CAD build for the part. Positions are in the model's coordinates, mm. A direction names the side the tool comes from. Coordinates: 2 decimals unless noted, no trailing zeros. Write each loop counter-clockwise with the first axis right and the second up, starting at its lowest first coordinate (ties: lowest second). Pieces come first, ordered by that corner, then holes. Notation, with made-up numbers: M -13,47 L 30,47 A16 cw 30,55 Z; hole C 27,57.25 d5. An arc over 180 degrees is marked long. Put each result on its own line as item: value. Start each with the question number.
Autodesk Inventor part; units mm, degrees
ref_plane "YZ Plane" through (0, 0, 0) normal (1, 0, 0) x (0, 1, 0)
ref_plane "XZ Plane" through (0, 0, 0) normal (0, 1, 0) x (-1, 0, 0)
ref_plane "XY Plane" through (0, 0, 0) normal (0, 0, 1) x (1, 0, 0)
sketch "Boceto1" plane through (0, 0, 0) normal (0, 1, 0) x (-1, 0, 0)
  circle A0 centre (0, 0) radius 37
  dimension "d0" = 74
extrude "Extrusión1" add sketch "Boceto1" along normal blind 11
sketch "Boceto3" plane through (0, 0, 0) normal (0, -1, 0) x (1, 0, 0)
  circle A0 centre (0, 0) radius 8.25
  circle A1 centre (0, 8.25) radius 1.7
  circle A2 centre (8.25, 0) radius 1.7
  circle A3 centre (-8.25, 0) radius 1.7
  circle A4 centre (0, -8.25) radius 1.7
  dimension "d7" = 3.4
  dimension "d8" = 16.5
extrude "Extrusión3" cut sketch "Boceto3" against normal through all contours A0 A2 | A0 A2 | A1 A0 | A0 A1 | A4 A0 | A0 A4 | A3 A0 | A0 A3
sketch "Boceto5" plane through (0, 0, 0) normal (0, -1, 0) x (1, 0, 0)
  circle A0 centre (0, 0) radius 4.05
  dimension "d13" = 8.1
extrude "Extrusión5" cut sketch "Boceto5" against normal through all
sketch "Boceto8" plane through (0, 11, 0) normal (0, 1, 0) x (1, 0, 0)
  circle A0 centre (0, 0) radius 24.5
  circle A1 centre (0, 0) radius 37
  dimension "d25" = 49
  dimension "d26" = 74
extrude "Extrusión8" cut sketch "Boceto8" against normal blind 4
sketch "Boceto14" plane through (0, 7, 0) normal (0, 1, 0) x (1, 0, 0)
  circle A0 centre (0, 0) radius 28
  circle A1 centre (0, 28) radius 1.7
  circle A2 centre (-24.2487, 14) radius 1.7
  circle A3 centre (-24.2487, -14) radius 1.7
  circle A4 centre (0, -28) radius 1.7
  circle A5 centre (24.2487, -14) radius 1.7
  circle A6 centre (24.2487, 14) radius 1.7
  point P0 (-1.6992, -27.9484)
  point P1 (1.6992, -27.9484)
  dimension "d50" = 56
  dimension "d51" = 3.4
  dimension "d54" = 360
extrude "Extrusión12" cut sketch "Boceto14" against normal through all contours A6 A0 | A0 A6 | A5 A0 | A0 A5 | A1 A0 | A0 A1 | A4 A0 | A0 A4 | A2 A0 | A0 A2 | A3 A0 | A0 A3
sketch "Boceto15" plane through (0, 7, 0) normal (0, 1, 0) x (1, 0, 0)
  circle A0 centre (24.2487, 14) radius 1.7
  circle A1 centre (24.2487, 14) radius 3
  circle A2 centre (0, 28) radius 3
  circle A3 centre (-24.2487, 14) radius 3
  circle A4 centre (-24.2487, -14) radius 3
  circle A5 centre (0, -28) radius 3
  circle A6 centre (24.2487, -14) radius 3
  circle A7 centre (0, 0) radius 4.05
  circle A8 centre (0, 0) radius 32.5
  circle A9 centre (0, 0) radius 24.5
  dimension "d58" = 6
  dimension "d61" = 360
  dimension "d63" = 65
extrude "Extrusión13" cut sketch "Boceto15" against normal blind 3 contours A0 | A1 | A2 | A3 | A4 | A5 | A6 | A8
sketch "Boceto16" plane through (0, 11, 0) normal (0, 1, 0) x (1, 0, 0)
  circle A0 centre (0, 0) radius 4.05
  circle A1 centre (0, 0) radius 14.5
  circle A2 centre (0, 0) radius 37
  dimension "d66" = 29
extrude "Extrusión14" cut sketch "Boceto16" against normal blind 4 contours A2
equation "\"d1\" = Altura"
equation "\"Altura\" = 11"
properties part number "Joint - Primer segmento" material "Plastico PETG"
(1) Slice it at C-C, the plane z = 28. Write the cut outline in (x, y).
(2) Slice it at A-A, the plane z = 0. Write the cut outline in (x, y), then the cut area to 3 significant figures.
(3) Slice it at D-D, the plane x = -8.25. Write the cut outline in (y, z).
(4) Drill centre lines: line 1 (Z direction, x = 0, y = 3.05); line 2 (X direction, y = 6.75, z = -7.5); line 3 (Z direction, x = 0, y = 6). Where is each one in solid material? Low to high. Write a range as [from, to].
(5) Two-plate mould, pull along Z, no slides. Class faces 3 (the face through (-3, 11, -3)), 4 (the face through (6.691, 9.028, 12.864)), 5 (the face through (-0.37, 5.42, -9.91)): +Z half, -Z half, draft (parallel to the pull), parting line (faces both ways), or undercut.
(6) Drop flat-ended pins along their axis: pin 1 (3 mm diameter, centred on x = 8, z = 24, fed in from +Y); pin 2 (6 mm diameter, centred on x = 25, z = 12, fed in from +Y); pin 3 (5 mm diameter, centred on y = 7.5, z = -11.5, fed in from -X); pin 4 (2 mm diameter, centred on x = 0, z = 28, fed in from -Y). Give the stop position or say it passes through.
(7) Slice it at B-B, the plane y = 2. State how many separate pieces and enclosed holes the cut face has, then the cut area to 3 significant figures.
(8) Which spindle directions (+Z, -Z, +X, -X, +Y, -Y) get a long thin tool onto all of the face, cutting with end or side? Do faces 1 (the face through (13.17, 5.52, -20.66)), 2 (the face through (-0.878, 5.423, -3.954)). Say none if no direction does.
Result set:
1. outline: M -24.19,0 L -1.7,0 L -1.7,4 L -16.5,4 L -16.5,7 L -24.19,7 Z; M 1.7,0 L 24.19,0 L 24.19,7 L 16.5,7 L 16.5,4 L 1.7,4 Z
2. outline: M -37,0 L -9.95,0 L -9.95,11 L -14.5,11 L -14.5,7 L -24.5,7 L -24.5,4 L -32.5,4 L -32.5,7 L -37,7 Z; M -6.55,0 L -4.05,0 L -4.05,11 L -6.55,11 Z; M 4.05,0 L 6.55,0 L 6.55,11 L 4.05,11 Z; M 9.95,0 L 37,0 L 37,7 L 32.5,7 L 32.5,4 L 24.5,4 L 24.5,7 L 14.5,7 L 14.5,11 L 9.95,11 Z
2. area: 422 mm^2
3. outline: M 0,-36.07 L 7,-36.07 L 7,-31.44 L 4,-31.44 L 4,-23.07 L 7,-23.07 L 7,-11.92 L 11,-11.92 L 11,-1.7 L 0,-1.7 Z; M 0,1.7 L 11,1.7 L 11,11.92 L 7,11.92 L 7,23.07 L 4,23.07 L 4,31.44 L 7,31.44 L 7,36.07 L 0,36.07 Z
4. line 1: z = [-37, -29.7], [-26.3, -9.95], [-6.55, -4.05], [4.05, 6.55], [9.95, 26.3], [29.7, 37]
4. line 2: x = [-36.23, -31.62], [-23.32, -1.53], [1.53, 23.32], [31.62, 36.23]
4. line 3: z = [-37, -32.5], [-24.5, -9.95], [-6.55, -4.05], [4.05, 6.55], [9.95, 24.5], [32.5, 37]
5. face 3: draft
5. face 4: parting line
5. face 5: undercut
6. pin 1: stops at y = 7
6. pin 2: stops at y = 4
6. pin 3: stops at x = -35.88
6. pin 4: passes through
7. separate pieces: 1
7. enclosed holes: 11
7. area: 4,160 mm^2
8. face 1: +Y
8. face 2: +Y, -Y
